Input: part model. Units: mm. Frame: model coordinates. A direction names the side the tool comes from. Coordinates: 2 decimals unless noted, no trailing zeros. Loops run counter-clockwise (first coordinate to the right, second up) from the corner with the lowest first, then second, coordinate; pieces in that order, holes last.
Autodesk Inventor part; units mm, degrees
ref_plane "Начальная плоскость" through (0, 0, 546.404) normal (0, 0, 1) x (1, 0, 0)
ref_plane "Конечная плоскость" through (0, 0, 696.459) normal (0, 0, 1) x (1, 0, 0)
ref_plane "РабПлоскость8" through (46, 32.5, 696.459) normal (0, 0, 1) x (1, 0, 0)
ref_plane "Начальная плоскость" through (0, 0, 546.404) normal (0, 0, 1) x (1, 0, 0)
ref_plane "Конечная плоскость" through (0, 0, 696.459) normal (0, 0, 1) x (1, 0, 0)
sketch "Эскиз" plane through (0, 0, 0) normal (0, 0, 1) x (1, 0, 0)
  line L0 (36, -32.5) -> (0, -32.5)
  line L1 (36, -32.5) -> (36, -28.696)
  line L2 (33.6994, -26.2039) -> (9.9215, -24.3017)
  line L3 (4.4, -18.3208) -> (4.4, 18.3208)
  line L4 (33.6994, 26.2039) -> (9.9215, 24.3017)
  line L5 (36, 28.696) -> (36, 32.5)
  line L6 (0, 32.5) -> (36, 32.5)
  line L7 (0, -32.5) -> (0, 32.5)
  arc A0 (4.4, -18.3208) -> (9.9215, -24.3017) centre (10.4, -18.3208) ccw
  arc A1 (9.9215, 24.3017) -> (4.4, 18.3208) centre (10.4, 18.3208) ccw
  arc A2 (36, -28.696) -> (33.6994, -26.2039) centre (33.5, -28.696) ccw
  arc A3 (33.6994, 26.2039) -> (36, 28.696) centre (33.5, 28.696) ccw
  line L8 (0, 45.5) -> (0, -45.5) construction
  line L9 (-7.2974, 0) -> (43.7847, 0) construction
  point P0 (36, -26.388)
  point P1 (4.4, -23.86)
  point P2 (4.4, 23.86)
  point P3 (36, 26.388)
  dimension "d3" = 36
  dimension "d5" = 4.4
  dimension "d7" = 65
  dimension "d9" = 8.64
  dimension "d11" = 8.64
  dimension "d13" = 6.112
  dimension "d15" = 6.112
  dimension "d22" = 6
  dimension "d23" = 2.5
  dimension "d24" = 32.5
  dimension "d25" = 0
extrude "Тело" add sketch "Эскиз" along normal up to surface (150.055 mm away) from surface at 546.404
sketch "Sketch3" plane through (0, 0, 0) normal (0, 0, 1) x (1, 0, 0)
  line L0 (0, 0) -> (10, 0)
ref_plane "Work Plane7" through (0, 0, 0) normal (0, -1, 0) x (1, 0, 0)
sketch "Sketch4" plane through (0, 0, 0) normal (0, -1, 0) x (1, 0, 0)
  line L0 (-2, 546.404) -> (12, 546.404)
  line L1 (-2, 696.459) -> (12, 696.459)
  dimension "d29" = 150.055
ref_plane "РабПлоскость8" through (46, 32.5, 696.459) normal (0, 0, 1) x (1, 0, 0)
split "Разделение1" plane through (46, 32.5, 696.459) removes the side toward (0, 0, 1)
ref_plane "РабПлоскость9" through (35.9999, -174.672, 546.4041) normal (0, 0, -1) x (-1, 0, 0)
split "Разделение2" plane through (35.9999, -174.672, 546.4041) removes the side toward (0, 0, -1)
equation "\"d3\" = b"
equation "\"d7\" = ParH"
equation "\"d22\" = R"
equation "\"d23\" = R1"
equation "\"d24\" = 0.5 * d7"
equation "\"d16\" = G_L"
equation "\"R1\" = 2.5"
equation "\"R\" = 6"
equation "\"t1\" = 4.4"
equation "\"t2\" = 7.2"
equation "\"ParH\" = 65"
equation "\"b\" = 36"
equation "\"msp_x1\" = 0.04 * b"
equation "\"msp_x2\" = -0.08 * t1 + 0.04 * b"
equation "\"G_L\" = d29"
equation "\"ex\" = 0"
equation "\"G_OFFSET_START\" = -546.404"
equation "\"d26\" = -G_OFFSET_START"
equation "\"d27\" = G_OFFSET_END + B_L"
equation "\"B_L\" = 796.459"
properties part number "Швеллер 6.5U-150,05 ГОСТ 8240-97" material "Сталь, мягкая"
Item 1: Section query D-D (y = 5.5). Output: boundary loops of the cut face in (x, z), then the cut area to 3 significant figures.
Result:
outline: (0, 546.4) - (4.4, 546.4) - (4.4, 696.46) - (0, 696.46) - close
area: 660 mm2
Item 2: Reachability of faces 1 (the face through (0, 0, 620)), 2 (the face through (21.977, -25.266, 620.381)) from +Z, -Z, +X, -X, +Y, -Y: full face, straight path, thin tool, end or side. Return the list, or none.
Result:
face 1: +Z, -Z, -X, +Y, -Y
face 2: +Z, -Z, +X
Item 3: Line query: L1, parallel to X at y = 12, z = 588.5; L2, parallel to Y at x = 8, z = 654; L3, parallel to Y at x = 21, z = 558.5. Output: solid intervals per line, ascending.
Result:
L1: x = 0 to 4.4
L2: y = -32.5 to -23.82, 23.82 to 32.5
L3: y = -32.5 to -25.19, 25.19 to 32.5
Item 4: Mould query, pull axis Y, two halves, no side actions, for faces 3 (the face through (3, 0, 696.459)), 4 (the face through (6, -22.4, 620.4)), 5 (the face through (18, -32.5, 620)). Classes: +Y half, -Y half, draft (parallel to the pull), parting line (faces both ways), or undercut.
Result:
face 3: draft
face 4: undercut
face 5: -Y half
Item 5: Section query C-C (x = 14). Output: boundary loops of the cut face in (y, z).
Result:
outline: (-32.5, 546.4) - (-24.63, 546.4) - (-24.63, 696.46) - (-32.5, 696.46) - close; (24.63, 546.4) - (32.5, 546.4) - (32.5, 696.46) - (24.63, 696.46) - close
Item 6: Contact query for flat-ended pins moving along their axis: P1, Ø5, axis at y = 1, z = 645.5, coming from the +X side; P2, Ø10, axis at x = 17.5, y = 21, coming from the +Z side. Output: stop coordinate, or through.
Result:
P1: stops at x = 4.4
P2: stops at z = 696.46
Item 7: Section query A-A (z = 624). Output: boundary loops of the cut face in (x, y).
Result:
outline: (0, -32.5) - (36, -32.5) - (36, -28.7) arc R2.5 ccw to (33.7, -26.2) - (9.92, -24.3) arc R6 cw to (4.4, -18.32) - (4.4, 18.32) arc R6 cw to (9.92, 24.3) - (33.7, 26.2) arc R2.5 ccw to (36, 28.7) - (36, 32.5) - (0, 32.5) - close
Item 8: Section query B-B (x = 6). Output: boundary loops of the cut face in (y, z).
Result:
outline: (-32.5, 546.4) - (-22.4, 546.4) - (-22.4, 696.46) - (-32.5, 696.46) - close; (22.4, 546.4) - (32.5, 546.4) - (32.5, 696.46) - (22.4, 696.46) - close
